```python
from build123d import *

# Parameters (mm, degrees)
BOSS_EXTRUDE1_DEPTH = 15
SKETCH2_R           = 7.5
BOSS_EXTRUDE2_DEPTH = 50
SCALE1_SCALE        = 10
SKETCH3_R           = 85
BOSS_EXTRUDE3_DEPTH = 20


with BuildPart() as part:
    # Sketch1 → Boss-Extrude1 (new body)
    with BuildSketch(Plane(origin=(0, 0, 0), x_dir=(1, 0, 0), z_dir=(0, 1, 0))):
        with BuildLine():
            Line((4.769696007, -1.5), (6, -1.5))
            Line((6, -1.5), (6, 1.5))
            Line((6, 1.5), (4.769696007, 1.5))
            ThreePointArc((4.769696007, 1.5), (-5, 0), (4.769696007, -1.5))
        make_face()
    extrude(amount=BOSS_EXTRUDE1_DEPTH)

    # Sketch2 → Boss-Extrude2 (add)
    with BuildSketch(Plane.XZ):
        with Locations(Location((0, 0, 0), (0, 0, 270))):
            Circle(SKETCH2_R)
    extrude(amount=BOSS_EXTRUDE2_DEPTH)


with BuildPart() as part_1:
    # Scale1: scaled about (0.026273948, -21.038472133, 0)
    add(part.part.scale(SCALE1_SCALE).moved(Location((-0.236465532, 189.346249197, 0))))

    # Sketch3 → Boss-Extrude3 (add)
    with BuildSketch(Plane(origin=(0, 189.346249199, 0), x_dir=(1, 0, 0), z_dir=(0, 1, 0))):
        with Locations(Location((0, 0, 0), (0, 0, 270))):
            Circle(SKETCH3_R)
    extrude(amount=-BOSS_EXTRUDE3_DEPTH)


solid = part_1.part
```
Here's how the part is built. I have some questions about the finished solid (model axes, mm). A direction names the side the tool comes from. Give positions to 0.01 mm unless a question says otherwise; leave off trailing zeros. Order: outer loops, then holes, each group sorted by start corner. A loop starts at its lowest first (then second) coordinate and runs counter-clockwise, first axis right, second up. Notation, with made-up numbers: M 63,48 L 107,48 A23 cw 107,64 Z; hole C 79.25,-3 d9. An arc over 180 degrees is marked long. Use a Markdown table: item, result. Add a question column.
1. For pin 1 Ø1 at (x, y) = (-30.5, 125.5) entering from +Z; pin 2 Ø6 at (x, y) = (-29, -126) entering from -Z; pin 3 Ø2 at (y, z) = (-182, -53) entering from -X, each with a flat end and sliding along its axis, tell me the tip position at first contact or that it passes through.
2. I need wall thicknesses on probe 1 along Y at (x, z) = (46.5, 21.5); probe 2 along X at (y, z) = (113.5, 2); probe 3 along Y at (x, z) = (52, 59.5). Which ranges of each line are inside material? Lowest first, please. Write a range as from..to.
3. Suppose I cut it at C-C (y = 207.5). List the corners of the cut face in (x, z) for me.
4. Suppose I cut it at B-B (x = 40.5). List the corners of the cut face in (y, z) for me.
5. On a 3-axis mill with a long thin cutter (end or side, diameter ignored), from which of +Z, -Z, +X, -X, +Y, -Y can I reach the whole of each face in a straight line? I mean faces 1 (the flat face through (59.764, 263, 0)), 2 (the flat face through (54, 263, -15)), 3 (the flat face through (-69, 169.346, 31)), 4 (the flat face through (54, 263, 15)). Say none if no direction works.
6. Suppose I cut it at A-A (z = 0). List the corners of the cut face in (x, y) for me, and give its area (3 significant figures).
7. Suppose I cut it at D-D (z = 57). List the corners of the cut face in (x, y) for me.
Results list:
| question | item | result |
|---|---|---|
| 1 | pin 1 | stops at z = 68.84 |
| 1 | pin 2 | stops at z = -70.44 |
| 1 | pin 3 | stops at x = -54.28 |
| 2 | probe 1 | y = -310.65..189.35 |
| 2 | probe 2 | x = -75.21..74.74 |
| 2 | probe 3 | y = 169.35..189.35 |
| 3 | outline | M 47.46,-15 L 59.76,-15 L 59.76,15 L 47.46,15 A50 ccw long Z |
| 4 | outline | M -310.65,-62.97 L 169.35,-62.97 L 169.35,-74.73 L 189.35,-74.73 L 189.35,-28.99 L 339.35,-28.99 L 339.35,28.99 L 189.35,28.99 L 189.35,74.73 L 169.35,74.73 L 169.35,62.97 L -310.65,62.97 Z |
| 5 | face 1 | +Z, -Z, +X, +Y |
| 5 | face 2 | -Z, +X, +Y |
| 5 | face 3 | -Y |
| 5 | face 4 | +Z, +X, +Y |
| 6 | outline | M -85,169.35 L -75.24,169.35 L -75.24,-310.65 L 74.76,-310.65 L 74.76,169.35 L 85,169.35 L 85,189.35 L 59.76,189.35 L 59.76,339.35 L -50.24,339.35 L -50.24,189.35 L -85,189.35 Z |
| 6 | area | 91,900 mm² |
| 7 | outline | M -63.06,169.35 L -48.98,169.35 L -48.98,-310.65 L 48.51,-310.65 L 48.51,169.35 L 63.06,169.35 L 63.06,189.35 L -63.06,189.35 Z |
